from build123d import *

# Parameters (mm, degrees)
SKETCH_1_W          = 29.8
SKETCH_1_H          = 29.8
SKETCH_1_W_2        = 25
SKETCH_1_H_2        = 25
EXTRUDE_1_DEPTH     = 40
CUT_EXTRUDE_1_REACH = 54.058
SKETCH_4_R          = 2.2
SKETCH_7_R          = 3.2
SKETCH_7_R_2        = 1.2
EXTRUDE_3_DEPTH     = 4
EXTRUDE_START       = -4
SKETCH_8_R          = 3.2
SKETCH_8_R_2        = 1.2
EXTRUDE_4_DEPTH     = 4
FILLET_2_R          = 10


with BuildPart() as part:
    # Эскиз1 → Вытянуть-Тонкостенный1 (new body)
    with BuildSketch(Plane(origin=(0, 0, 0), x_dir=(0, 0, -1), z_dir=(1, 0, 0))):
        Rectangle(SKETCH_1_W, SKETCH_1_H)
        Rectangle(SKETCH_1_W_2, SKETCH_1_H_2, mode=Mode.SUBTRACT)
    extrude(amount=EXTRUDE_1_DEPTH)

    # Эскиз4 → Вырез-Вытянуть1 (cut, up to next)
    with BuildSketch(Plane(origin=(0, 14.9, 0), x_dir=(1, 0, 0), z_dir=(0, 1, 0)), mode=Mode.PRIVATE) as cut_extrude_1_sk1:
        with Locations(Location((20, 0, 0), (0, 0, 270))):
            Circle(SKETCH_4_R)
    cut_extrude_1_tool1 = extrude(cut_extrude_1_sk1.sketch, amount=-CUT_EXTRUDE_1_REACH, mode=Mode.PRIVATE) & part.part
    add(cut_extrude_1_tool1.solids().sort_by_distance((20, 14.9, 0))[0], mode=Mode.SUBTRACT)

    # Эскиз7 → Бобышка-Вытянуть3 (add)
    with BuildSketch(Plane.XZ.offset(14.9)):
        with Locations((20, -17.9)):
            Circle(SKETCH_7_R)
        with Locations(Location((20, -17.9, 0), (0, 0, 270))):
            Circle(SKETCH_7_R_2, mode=Mode.SUBTRACT)
    extrude(amount=-EXTRUDE_3_DEPTH)

    # Эскиз8 → Бобышка-Вытянуть4 (add)
    with BuildSketch(Plane(origin=(0, 14.9, 0), x_dir=(1, 0, 0), z_dir=(0, 1, 0)).offset(EXTRUDE_START)):
        with Locations((20, 17.9)):
            Circle(SKETCH_8_R)
        with Locations(Location((20, 17.9, 0), (0, 0, 90))):
            Circle(SKETCH_8_R_2, mode=Mode.SUBTRACT)
    extrude(amount=EXTRUDE_4_DEPTH)

    # Скругление2
    fillet_2_edges = [part.edges().sort_by_distance(p)[0] for p in [
        (18.886447127, -12.9, -14.9),
        (21.113552873, -12.9, -14.9),
        (21.113552873, 12.9, -14.9),
        (18.886447127, 12.9, -14.9),
    ]]
    fillet(fillet_2_edges, radius=FILLET_2_R)


solid = part.part
Work out the finished part from the listing and answer in its coordinate system (mm). A direction names the side the tool comes from. Round coordinates to 2 decimals unless told otherwise and drop trailing zeros. Write each loop counter-clockwise with the first axis right and the second up, starting at its lowest first coordinate (ties: lowest second). Pieces come first, ordered by that corner, then holes. Notation, with made-up numbers: (-24.5, -15) - (23.5, -15) arc R21 cw to (23.5, 1) - close; hole circle Ø6 at (51.5, 76). An arc over 180 degrees is marked (long way). Answer in a Markdown table with one row per item. Add a question column.
1. A cutting plane is placed at A-A, the plane x = 20. Determine the outline of the cut face in (y, z).
2. Given pin 1 (1.4 mm diameter, centred on x = 20, z = -17.9, fed in from -Y); pin 2 (3 mm diameter, centred on x = 33, y = -3, fed in from -Z); pin 3 (4 mm diameter, centred on x = 20, z = 0, fed in from +Y), each flat-ended and moving along its own axis, determine where each tip first touches the part or whether it passes through.
3. A cutting plane is placed at B-B, the plane z = -11. Determine the outline of the cut face in (x, y).
4. The mould has two halves that part along Y. Classify faces 4 (the flat face through (20, 14.9, -3)), 5 (the cylindrical face through (17.852, 13.717, -0.477)), 6 (the flat face through (20, -12.5, 0)): +Y half, -Y half, draft (parallel to the pull), parting line (faces both ways), or undercut.
5. Find the intervals of material crossed by line 1 along Y through (x, z) = (37, -4); line 2 along X through (y, z) = (13.8, 0), in increasing order. Write a range as from..to.
6. A cutting plane is placed at D-D, the plane z = 0. Determine the outline of the cut face in (x, y), and give its area (3 significant figures).
7. For faces 1 (the flat face through (20, -10.9, -16)), 2 (the cylindrical face through (20, -12.9, -21.1)), 3 (the flat face through (20, 12.5, 3)), determine the directions among +Z, -Z, +X, -X, +Y, -Y from which every point of the face is accessible in a straight line to the end or side of a thin tool.
Worked out:
| question | item | result |
|---|---|---|
| 1 | outline | (-14.9, -21.1) - (-10.9, -21.1) - (-10.9, -19.1) - (-14.9, -19.1) - close; (-14.9, -16.7) - (-10.9, -16.7) - (-10.9, -14.9) - (10.9, -14.9) - (10.9, -16.7) - (14.9, -16.7) - (14.9, -2.2) - (12.5, -2.2) - (12.5, -12.5) - (-12.5, -12.5) - (-12.5, 12.5) - (12.5, 12.5) - (12.5, 2.2) - (14.9, 2.2) - (14.9, 14.9) - (-14.9, 14.9) - close; (10.9, -21.1) - (14.9, -21.1) - (14.9, -19.1) - (10.9, -19.1) - close |
| 2 | pin 1 | through |
| 2 | pin 2 | z = -14.9 |
| 2 | pin 3 | y = -12.5 |
| 3 | outline | (0, -14.9) - (40, -14.9) - (40, -12.5) - (0, -12.5) - close; (0, 12.5) - (40, 12.5) - (40, 14.9) - (0, 14.9) - close |
| 4 | face 4 | +Y half |
| 4 | face 5 | draft |
| 4 | face 6 | undercut |
| 5 | line 1 | -14.9..-12.5, 12.5..14.9 |
| 5 | line 2 | 0..17.8, 22.2..40 |
| 6 | outline | (0, -14.9) - (40, -14.9) - (40, -12.5) - (0, -12.5) - close; (0, 12.5) - (17.8, 12.5) - (17.8, 14.9) - (0, 14.9) - close; (22.2, 12.5) - (40, 12.5) - (40, 14.9) - (22.2, 14.9) - close |
| 6 | area | 181 mm^2 |
| 7 | face 1 | -Z, +X, -X |
| 7 | face 2 | -Z, +Y, -Y |
| 7 | face 3 | +X, -X |
